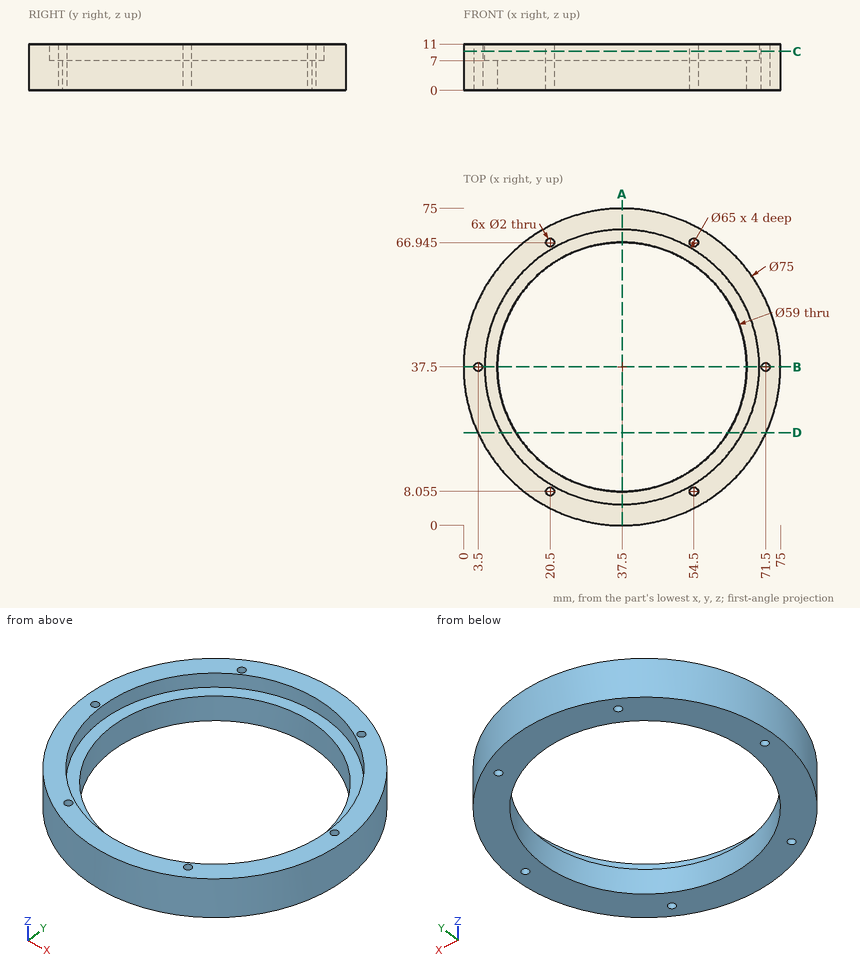
For this review, use the dimensioned drawing (mm, ordinates from the lowest corner) and the shaded views. Give positions to 0.01 mm unless a question says otherwise; leave off trailing zeros. Loops run counter-clockwise (first coordinate to the right, second up) from the corner with the lowest first, then second, coordinate; pieces in that order, holes last. Notation, with made-up numbers: (-6.75, 41.5) -> (-2.75, 41.5) arc R24 ccw to (-2.75, 63.5) -> close; hole circle Ø8 at (15, 32.25). An arc over 180 degrees is marked (long way). One line per question, with ' | ' between items. Start each with the question number.
(1) We need section B-B (y = 37.5). State the section outline as (x, z) points, and give its area (3 significant figures).
(2) We need section A-A (x = 37.5). State the section outline as (y, z) points.
(3) We need section D-D (y = 22). State the section outline as (x, z) points.
(4) For line 1 (Y direction, x = 37.5, z = 3.5); line 2 (Y direction, x = 20.5, z = 5.75) (1 decimal); line 3 (X direction, y = 37, z = 8.25), list the stretches that pass through material, from the lowest coordinate up.
(5) We need section C-C (z = 9.25). State the section outline as (x, y) points (3 decimals).
(6) Insertion check: P1, Ø2.5, axis at x = 20.5, y = 8.06, coming from the +Z side; P2, Ø1.5, axis at y = 49, z = 6.5, coming from the +X side; P3, Ø3, axis at y = 18, z = 8.5, coming from the -X side; P4, Ø3, axis at x = 17, z = 3, coming from the +Y side. Each pin has a flat end and moves straight along its axis. Give the tip position at first contact, or say it passes through.
The answers:
1) outline: (0, 0) -> (2.5, 0) -> (2.5, 11) -> (0, 11) -> close; (4.5, 0) -> (8, 0) -> (8, 7) -> (5, 7) -> (5, 11) -> (4.5, 11) -> close; (67, 0) -> (70.5, 0) -> (70.5, 11) -> (70, 11) -> (70, 7) -> (67, 7) -> close; (72.5, 0) -> (75, 0) -> (75, 11) -> (72.5, 11) -> close | area: 108 mm^2
2) outline: (0, 0) -> (8, 0) -> (8, 7) -> (5, 7) -> (5, 11) -> (0, 11) -> close; (67, 0) -> (75, 0) -> (75, 11) -> (70, 11) -> (70, 7) -> (67, 7) -> close
3) outline: (3.35, 0) -> (12.4, 0) -> (12.4, 7) -> (8.93, 7) -> (8.93, 11) -> (3.35, 11) -> close; (62.6, 0) -> (71.65, 0) -> (71.65, 11) -> (66.07, 11) -> (66.07, 7) -> (62.6, 7) -> close
4) line 1: y = 0 to 8, 67 to 75 | line 2: y = 4.1 to 7.1, 9.1 to 13.4, 61.6 to 65.9, 67.9 to 70.9 | line 3: x = 0 to 2.63, 4.37 to 5, 70 to 70.63, 72.37 to 75
5) outline: circle Ø75 at (37.5, 37.5); hole circle Ø2 at (3.5, 37.5); hole circle Ø65 at (37.5, 37.5); hole circle Ø2 at (20.5, 8.055); hole circle Ø2 at (20.5, 66.945); hole circle Ø2 at (54.5, 8.055); hole circle Ø2 at (54.5, 66.945); hole circle Ø2 at (71.5, 37.5)
6) P1: stops at z = 11 | P2: stops at x = 73.43 | P3: stops at x = 4.6 | P4: stops at y = 69.83
